from build123d import *

# Parameters (mm, degrees)
F1_DEPTH = 50
F2_DEPTH = 25


with BuildPart() as f1:
    # F0 (on Front) → F1 (new body)
    with BuildSketch(Plane.XZ):
        with BuildLine():
            ThreePointArc((191.0551849335, -10), (183.9841171217, -7.0710678119), (181.0551849335, 0))
            ThreePointArc((181.0551849335, 0), (181.2071074034, 1.7364817767), (181.6582587257, 3.4202014333))
            Line((181.6582587257, 3.4202014333), (184.0531095514, 10))
            Line((184.0531095514, 10), (0, 10))
            ThreePointArc((0, 10), (-10, 0), (0, -10))
            Line((0, -10), (191.0551849335, -10))
        make_face()
        with BuildLine():
            ThreePointArc((122.5, 0), (120, -2.5), (117.5, 0))
            ThreePointArc((117.5, 0), (120, 2.5), (122.5, 0))
        make_face(mode=Mode.SUBTRACT)
        with BuildLine():
            Line((191.0551849335, 0), (181.0551849335, 0))
            ThreePointArc((181.0551849335, 0), (183.9841171217, -7.0710678119), (191.0551849335, -10))
            ThreePointArc((191.0551849335, -10), (196.790949297, -8.1915204429), (200.4521111414, -3.4202014333))
            ThreePointArc((200.4521111414, -3.4202014333), (200.1182628039, 4.2261826174), (194.4753863668, 9.3969262079))
            Line((194.4753863668, 9.3969262079), (191.0551849335, 0))
        make_face()
        with BuildLine():
            ThreePointArc((191.0551849335, 10), (192.7916667102, 9.8480775301), (194.4753863668, 9.3969262079))
            ThreePointArc((194.4753863668, 9.3969262079), (200.1182628039, 4.2261826174), (200.4521111414, -3.4202014333))
            Line((200.4521111414, -3.4202014333), (239.3969262079, 103.5797985667))
            ThreePointArc((239.3969262079, 103.5797985667), (233.4202014333, 116.3969262079), (220.6030737921, 110.4202014333))
            Line((220.6030737921, 110.4202014333), (184.0531095514, 10))
            Line((184.0531095514, 10), (191.0551849335, 10))
        make_face()
        with BuildLine():
            ThreePointArc((232.5, 107), (231.4339410909, 104.9521198893), (229.1449496417, 104.650768448))
            ThreePointArc((229.1449496417, 104.650768448), (228.5660589091, 109.0478801107), (232.5, 107))
        make_face(mode=Mode.SUBTRACT)
        with BuildLine():
            ThreePointArc((181.6582587257, 3.4202014333), (181.2071074034, 1.7364817767), (181.0551849335, 0))
            Line((181.0551849335, 0), (191.0551849335, 0))
            Line((191.0551849335, 0), (194.4753863668, 9.3969262079))
            ThreePointArc((194.4753863668, 9.3969262079), (192.7916667102, 9.8480775301), (191.0551849335, 10))
            Line((191.0551849335, 10), (184.0531095514, 10))
            Line((184.0531095514, 10), (181.6582587257, 3.4202014333))
        make_face()
        with BuildLine():
            ThreePointArc((232.5, 107), (228.5660589091, 109.0478801107), (229.1449496417, 104.650768448))
            ThreePointArc((229.1449496417, 104.650768448), (231.4339410909, 104.9521198893), (232.5, 107))
        make_face()
        with BuildLine():
            Line((122.5, 0), (117.5, 0))
            ThreePointArc((117.5, 0), (120, -2.5), (122.5, 0))
        make_face()
        with BuildLine():
            ThreePointArc((122.5, 0), (120, 2.5), (117.5, 0))
            Line((117.5, 0), (122.5, 0))
        make_face()
    extrude(amount=F1_DEPTH)

    # F0 (on Front) → F2 (cut)
    with BuildSketch(Plane.XZ):
        with BuildLine():
            ThreePointArc((191.0551849335, -10), (183.9841171217, -7.0710678119), (181.0551849335, 0))
            ThreePointArc((181.0551849335, 0), (181.2071074034, 1.7364817767), (181.6582587257, 3.4202014333))
            Line((181.6582587257, 3.4202014333), (184.0531095514, 10))
            Line((184.0531095514, 10), (0, 10))
            ThreePointArc((0, 10), (-10, 0), (0, -10))
            Line((0, -10), (191.0551849335, -10))
        make_face()
        with BuildLine():
            ThreePointArc((122.5, 0), (120, -2.5), (117.5, 0))
            ThreePointArc((117.5, 0), (120, 2.5), (122.5, 0))
        make_face(mode=Mode.SUBTRACT)
        with BuildLine():
            ThreePointArc((181.6582587257, 3.4202014333), (181.2071074034, 1.7364817767), (181.0551849335, 0))
            Line((181.0551849335, 0), (191.0551849335, 0))
            Line((191.0551849335, 0), (194.4753863668, 9.3969262079))
            ThreePointArc((194.4753863668, 9.3969262079), (192.7916667102, 9.8480775301), (191.0551849335, 10))
            Line((191.0551849335, 10), (184.0531095514, 10))
            Line((184.0531095514, 10), (181.6582587257, 3.4202014333))
        make_face()
        with BuildLine():
            Line((191.0551849335, 0), (181.0551849335, 0))
            ThreePointArc((181.0551849335, 0), (183.9841171217, -7.0710678119), (191.0551849335, -10))
            ThreePointArc((191.0551849335, -10), (196.790949297, -8.1915204429), (200.4521111414, -3.4202014333))
            ThreePointArc((200.4521111414, -3.4202014333), (200.1182628039, 4.2261826174), (194.4753863668, 9.3969262079))
            Line((194.4753863668, 9.3969262079), (191.0551849335, 0))
        make_face()
        with BuildLine():
            ThreePointArc((191.0551849335, 10), (192.7916667102, 9.8480775301), (194.4753863668, 9.3969262079))
            ThreePointArc((194.4753863668, 9.3969262079), (200.1182628039, 4.2261826174), (200.4521111414, -3.4202014333))
            Line((200.4521111414, -3.4202014333), (239.3969262079, 103.5797985667))
            ThreePointArc((239.3969262079, 103.5797985667), (233.4202014333, 116.3969262079), (220.6030737921, 110.4202014333))
            Line((220.6030737921, 110.4202014333), (184.0531095514, 10))
            Line((184.0531095514, 10), (191.0551849335, 10))
        make_face()
        with BuildLine():
            ThreePointArc((232.5, 107), (231.4339410909, 104.9521198893), (229.1449496417, 104.650768448))
            ThreePointArc((229.1449496417, 104.650768448), (228.5660589091, 109.0478801107), (232.5, 107))
        make_face(mode=Mode.SUBTRACT)
    extrude(amount=F2_DEPTH, mode=Mode.SUBTRACT)

    # F3: F1 across plane


with BuildPart() as f1_1:
    add(f1.part)
    add(f1.part.mirror(Plane.YZ))


with BuildPart() as f4_1:
    # F4: copy of F1
    add(f1_1.part)


solid = f1_1.part
Can you work these out from the model? Positions are in its coordinate system, mm. A direction names the side the tool comes from. Coordinates: 2 decimals unless noted, no trailing zeros. Order: outer loops, then holes, each group sorted by start corner. A loop starts at its lowest first (then second) coordinate and runs counter-clockwise, first axis right, second up. Notation, with made-up numbers: (53, 45.25) - (105, 45.25) arc R22 ccw to (105, 56.25) - close; hole circle Ø2 at (-2, -28.5). An arc over 180 degrees is marked (long way). Answer as a JSON object with one key per item and string values. Group by question number.
Q1. Imagine slicing it at A-A (z = 75.5). Please give me the cut outline in (x, y).
Q2. I need wall thicknesses on line 1 (Z direction, x = 164, y = -35); line 2 (Y direction, x = 216.5, z = 69.5); line 3 (X direction, y = -41, z = 6). Which ranges of each line are inside material? Lowest first, please. Write a range as from..to.
Q3. Will these pins go through, and if not, where does the flat tip stop? P1, Ø3, axis at y = -43.5, z = 15, coming from the +X side; P2, Ø1.5, axis at y = -37.5, z = 51, coming from the +X side; P3, Ø12.5, axis at x = -57.5, y = -40.5, coming from the +Z side.
Q4. Imagine slicing it at B-B (y = -19). Please give me the cut outline in (x, z).
Q5. Imagine slicing it at C-C (x = 79). Please give me the cut outline in (y, z).
Q6. On a 3-axis mill with a long thin cutter (end or side, diameter ignored), from which of +Z, -Z, +X, -X, +Y, -Y can I reach the whole of each face in a straight line? I mean faces 1 (the face through (202.584, -37.325, 60.913)), 2 (the face through (-219.65, -37.33, 49.33)). Say none if no direction works.
Determined:
{
 "1": {"outline": "(-229.18, -50) - (-207.89, -50) - (-207.89, -25) - (-229.18, -25) - close; (207.89, -50) - (229.18, -50) - (229.18, -25) - (207.89, -25) - close"},
 "2": {"line 1": "z = -10..10", "line 2": "y = -50..-25", "line 3": "x = -203.88..203.88"},
 "3": {"P1": "stops at x = 207.7", "P2": "stops at x = 220.53", "P3": "stops at z = 10"},
 "4": {"outline": "circle Ø5 at (-230, 107); circle Ø5 at (-120, 0); circle Ø5 at (120, 0); circle Ø5 at (230, 107)"},
 "5": {"outline": "(-50, -10) - (-25, -10) - (-25, 10) - (-50, 10) - close"},
 "6": {"face 1": "+Z, +Y, -Y", "face 2": "-Z, -X, +Y, -Y"}
}
